Source: three-view drawing plus pictorial views. Frame: mm from the lowest corner of the part. Give positions to 0.01 mm unless a question says otherwise; leave off trailing zeros. Order: outer loops, then holes, each group sorted by start corner. A loop starts at its lowest first (then second) coordinate and runs counter-clockwise, first axis right, second up.
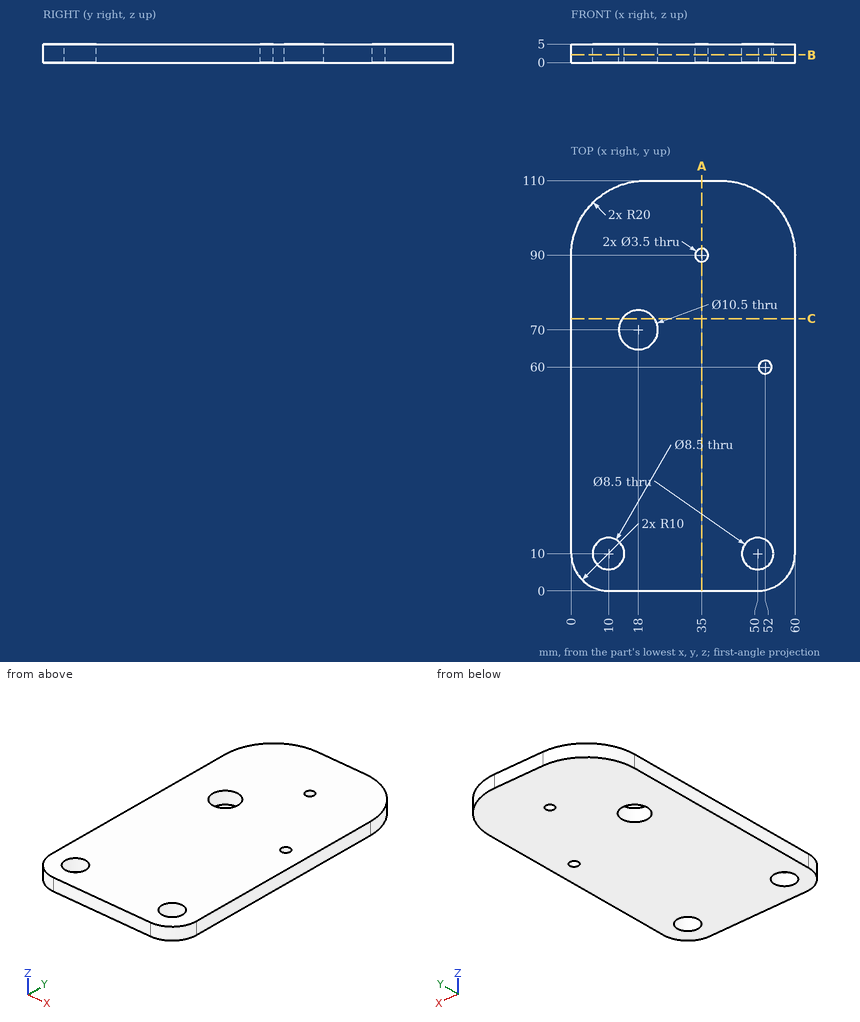
1) Section query C-C on y = 73. Output: boundary loops of the cut face in (x, z), and give its area (3 significant figures).
Checks:
outline: (0, 0) - (13.69, 0) - (13.69, 5) - (0, 5) - close; (22.31, 0) - (60, 0) - (60, 5) - (22.31, 5) - close
area: 257 mm2
2) Section query B-B on z = 2.1. Output: boundary loops of the cut face in (x, y).
Checks:
outline: (0, 10) arc R10 ccw to (10, 0) - (50, 0) arc R10 ccw to (60, 10) - (60, 90) arc R20 ccw to (40, 110) - (20, 110) arc R20 ccw to (0, 90) - close; hole circle Ø8.5 at (10, 10); hole circle Ø10.5 at (18, 70); hole circle Ø3.5 at (35, 90); hole circle Ø8.5 at (50, 10); hole circle Ø3.5 at (52, 60)
3) Section query A-A on x = 35. Output: boundary loops of the cut face in (y, z).
Checks:
outline: (0, 0) - (88.25, 0) - (88.25, 5) - (0, 5) - close; (91.75, 0) - (110, 0) - (110, 5) - (91.75, 5) - close
4) Ray query, L1, parallel to Y at x = 13.5, z = 3.15; L2, parallel to X at y = 69.5, z = 0.45; L3, parallel to X at y = 90, z = 3.1. Return the intervals inside material, ascending.
Checks:
L1: y = 0 to 7.59, 12.41 to 67.3, 72.7 to 108.91
L2: x = 0 to 12.77, 23.23 to 60
L3: x = 0 to 33.25, 36.75 to 60
